Geometry check sheet. Reference: the model listing, model coordinates, mm. A direction names the side the tool comes from. Round coordinates to 2 decimals unless told otherwise and drop trailing zeros. Write each loop counter-clockwise with the first axis right and the second up, starting at its lowest first coordinate (ties: lowest second). Pieces come first, ordered by that corner, then holes. Notation, with made-up numbers: (37.5, 88) -> (61.5, 88) arc R24 cw to (61.5, 108) -> close; hole circle Ø4 at (43, 51). An arc over 180 degrees is marked (long way). Use a Markdown table: item, result.
Autodesk Inventor part; units mm, degrees
ref_plane "YZ Plane" through (0, 0, 0) normal (1, 0, 0) x (0, 1, 0)
ref_plane "XZ Plane" through (0, 0, 0) normal (0, 1, 0) x (-1, 0, 0)
ref_plane "XY Plane" through (0, 0, 0) normal (0, 0, 1) x (1, 0, 0)
sketch "Sketch1" plane through (0, 0, 0) normal (0, 0, 1) x (1, 0, 0)
  circle A0 centre (0, 0) radius 9
  dimension "d0" = 18
extrude "Extrusion1" add sketch "Sketch1" along normal blind 1
sketch "Sketch2" plane through (0, 0, 1) normal (0, 0, 1) x (1, 0, 0)
  circle A0 centre (0, 0) radius 9
  circle A1 centre (0, 0) radius 8
  dimension "d4" = 16
extrude "Extrusion2" add sketch "Sketch2" along normal blind 4 contours A1
sketch "Sketch3" plane through (0, 0, 5) normal (0, 0, 1) x (1, 0, 0)
  circle A0 centre (0, 0) radius 8
  circle A1 centre (0, 0) radius 2.5
  dimension "d8" = 5
extrude "Extrusion3" cut sketch "Sketch3" against normal through all contours A1
properties part number "f625"
(1) Section check D-D on x = 7.25. Record the cut outline in (y, z).
A:
| item | result |
|---|---|
| outline | (-5.33, 0) -> (5.33, 0) -> (5.33, 1) -> (3.38, 1) -> (3.38, 5) -> (-3.38, 5) -> (-3.38, 1) -> (-5.33, 1) -> close |
(2) Section check A-A on y = 0. Record the cut outline in (x, z).
A:
| item | result |
|---|---|
| outline | (-9, 0) -> (-2.5, 0) -> (-2.5, 5) -> (-8, 5) -> (-8, 1) -> (-9, 1) -> close; (2.5, 0) -> (9, 0) -> (9, 1) -> (8, 1) -> (8, 5) -> (2.5, 5) -> close |
(3) Release check for a two-part mould opening along X. For faces 3 (the face through (-0.54, -2.44, 2.54)), 4 (the face through (-2, -2, 5)), 5 (the face through (-1.172, -8.923, 0.493)) record: +X half, -X half, draft (parallel to the pull), parting line (faces both ways), or undercut.
A:
| item | result |
|---|---|
| face 3 | undercut |
| face 4 | draft |
| face 5 | parting line |
(4) Thickness scan on line 1 (Y direction, x = 0, z = 3.2); line 2 (Y direction, x = 1, z = 3.55); line 3 (Z direction, x = -7.25, y = -3.5). Record the ranges inside material, lowest first.
A:
| item | result |
|---|---|
| line 1 | y = -8 to -2.5, 2.5 to 8 |
| line 2 | y = -7.94 to -2.29, 2.29 to 7.94 |
| line 3 | z = 0 to 1 |
(5) Gauge pin test, flat ends, axial feed: pin 1 Ø3 at (x, z) = (1, 3) entering from -Y; pin 2 Ø2 at (y, z) = (5, 3.5) entering from -X; pin 3 Ø1.5 at (y, z) = (-5.5, 1) entering from -X. Record the tip position at first contact, or that the pin passes through.
A:
| item | result |
|---|---|
| pin 1 | stops at y = -8 |
| pin 2 | stops at x = -6.93 |
| pin 3 | stops at x = -7.64 |
(6) Section check C-C on y = -3. Record the cut outline in (x, z), plus the area to 3 significant figures.
A:
| item | result |
|---|---|
| outline | (-8.49, 0) -> (8.49, 0) -> (8.49, 1) -> (7.42, 1) -> (7.42, 5) -> (-7.42, 5) -> (-7.42, 1) -> (-8.49, 1) -> close |
| area | 76.3 mm2 |
(7) Access from +Z, -Z, +X, -X, +Y, -Y to the whole of each face (thin tool, end or side, straight path). Record for faces 1 (the face through (2, -2, 0)), 2 (the face through (-1.73, 7.81, 2.97)).
A:
| item | result |
|---|---|
| face 1 | -Z, +X, -X, +Y, -Y |
| face 2 | +Z |
